CAD build for the part. Positions are in the model's coordinates, mm. A direction names the side the tool comes from. Coordinates: 2 decimals unless noted, no trailing zeros. Order: outer loops, then holes, each group sorted by start corner. A loop starts at its lowest first (then second) coordinate and runs counter-clockwise, first axis right, second up. Notation, with made-up numbers: M 33.25,-30.75 L 79.25,-30.75 A20 ccw 79.25,0.25 Z; hole C 48.5,26.5 d4. An arc over 180 degrees is marked long. One line per item, written item: value.
from build123d import *

# Parameters (mm, degrees)
BOSS_EXTRUDE1_DEPTH     = 100
BOSS_EXTRUDE2_DEPTH     = 100
CUT_EXTRUDE1_DEPTH      = 10
CHAMFER1_SIZE           = 5.5
CHAMFER2_SIZE           = 4
SKETCH8_R               = 2
BOSS_EXTRUDE3_DEPTH     = 9.3
CUT_EXTRUDE3_DEPTH      = 125.214315536
CUT_EXTRUDE3_DEPTH_BACK = 10
SKETCH9_W               = 11
SKETCH9_H               = 9.3
CHAMFER3_SIZE           = 4
CHAMFER4_SIZE           = 3
CHAMFER5_SIZE           = 3
SKETCH10_W              = 5
SKETCH10_H              = 10
CUT_EXTRUDE4_DEPTH      = 94
CHAMFER7_SIZE           = 1
CHAMFER8_SIZE           = 1
SKETCH11_R              = 2.05
CUT_EXTRUDE5_DEPTH      = 10
CHAMFER9_SIZE           = 0.5
SKETCH12_R              = 2
CUT_EXTRUDE6_DEPTH      = 15
SKETCH20_W              = 62.3
SKETCH20_H              = 63.674798271
CUT_EXTRUDE14_DEPTH     = 15
BOSS_EXTRUDE4_DEPTH     = 6
SKETCH22_R              = 2
CUT_EXTRUDE15_DEPTH     = 10
CHAMFER10_SIZE          = 1
CHAMFER10_SIZE2         = 0.414213562
CHAMFER11_SIZE          = 1
CHAMFER11_SIZE2         = 0.414213562


with BuildPart() as part:
    # Sketch4 → Boss-Extrude1 (new body)
    with BuildSketch(Plane.XY):
        Polygon((-18.358738987, 4.974798271), (-27, 4.974798271), (-27, -6.2), (27, -6.2), (27, 4.974798271), (18.358738987, 4.974798271), (21.346410162, -0.2), (-21.346410162, -0.2), align=None)
    extrude(amount=BOSS_EXTRUDE1_DEPTH)

    # Sketch6 → Boss-Extrude2 (add)
    with BuildSketch(Plane.XY.offset(100)):
        Polygon((-24.15, 4.974798271), (-24.15, 52.474798271), (-5.5, 52.474798271), (-5.5, 57.474798271), (-31.15, 57.474798271), (-31.15, -6.2), (-24.15, -6.2), align=None)
        Polygon((24.15, -6.2), (24.15, 52.474798271), (5.5, 52.474798271), (5.5, 57.474798271), (31.15, 57.474798271), (31.15, -6.2), align=None)
    extrude(amount=-BOSS_EXTRUDE2_DEPTH)

    # Sketch7 → Cut-Extrude1 (cut)
    with BuildSketch(Plane(origin=(31.15, 0, 0), x_dir=(0, 0, -1), z_dir=(1, 0, 0))):
        Polygon((-85, 28.724798271), (-81.5, 25.224798271), (-13.5, 25.224798271), (-10, 28.724798271), (-13.5, 32.224798271), (-81.5, 32.224798271), align=None)
    extrude(amount=-CUT_EXTRUDE1_DEPTH, mode=Mode.SUBTRACT)

    # Chamfer1
    chamfer1_edges = [part.edges().sort_by_distance(p)[0] for p in [
        (-24.15, 52.474798271, 50),
        (-24.15, 4.974798271, 50),
        (24.15, 4.974798271, 50),
        (24.15, 52.474798271, 50),
    ]]
    chamfer(chamfer1_edges, length=CHAMFER1_SIZE)

    # Chamfer2
    chamfer2_edges = [part.edges().sort_by_distance(p)[0] for p in [
        (-5.5, 52.474798271, 50),
        (5.5, 52.474798271, 50),
    ]]
    chamfer(chamfer2_edges, length=CHAMFER2_SIZE)

    # Sketch8 → Boss-Extrude3 (add)
    with BuildSketch(Plane(origin=(0, 57.474798271, 0), x_dir=(1, 0, 0), z_dir=(0, 1, 0))):
        Polygon((-21.8, -70), (13.8, -70), (21.8, -62), (21.8, -14), (13.8, -6), (-21.8, -6), align=None)
        with Locations(Location((9.8, -62, 0), (0, 0, 270))):
            Circle(SKETCH8_R, mode=Mode.SUBTRACT)
        with Locations(Location((11.8, -14, 0), (0, 0, 270))):
            Circle(SKETCH8_R, mode=Mode.SUBTRACT)
        with Locations(Location((-11.8, -14, 0), (0, 0, 270))):
            Circle(SKETCH8_R, mode=Mode.SUBTRACT)
        with Locations(Location((-9.8, -62, 0), (0, 0, 270))):
            Circle(SKETCH8_R, mode=Mode.SUBTRACT)
    extrude(amount=BOSS_EXTRUDE3_DEPTH)

    # Sketch9 → Cut-Extrude3 (cut, two sides: drawn at the far end of the back side and taken through both)
    with BuildSketch(Plane.XY.offset(-CUT_EXTRUDE3_DEPTH_BACK)):
        with Locations((0, 62.124798271)):
            Rectangle(SKETCH9_W, SKETCH9_H)
    extrude(amount=CUT_EXTRUDE3_DEPTH + CUT_EXTRUDE3_DEPTH_BACK, mode=Mode.SUBTRACT)

    # Chamfer3
    chamfer3_edges = [part.edges().sort_by_distance(p)[0] for p in [
        (-31.15, -6.2, 50),
        (-31.15, 57.474798271, 50),
        (31.15, -6.2, 50),
        (31.15, 57.474798271, 50),
    ]]
    chamfer(chamfer3_edges, length=CHAMFER3_SIZE)

    # Chamfer4
    chamfer4_edges = [part.edges().sort_by_distance(p)[0] for p in [
        (9.65, 57.474798271, 70),
        (-21.8, 57.474798271, 38),
        (-13.65, 57.474798271, 70),
        (17.8, 57.474798271, 66),
        (21.8, 57.474798271, 38),
        (17.8, 57.474798271, 10),
        (9.65, 57.474798271, 6),
        (-13.65, 57.474798271, 6),
    ]]
    chamfer(chamfer4_edges, length=CHAMFER4_SIZE)

    # Chamfer5
    # the kernel refuses this chamfer: 3 mm, written as the material it adds along each edge
    with BuildSketch(Plane(origin=(31.15, 25.224798271, 81.5), x_dir=(0, -0.014760203742521738, -0.9998910622590239), z_dir=(-1, 0, 0)), Plane(origin=(31.15, 32.224798271, 81.5), x_dir=(0, -0.6965927104131427, 0.7174667907292097), z_dir=(-1, 0, 0))) as chamfer5_piece_1:
        Polygon((CHAMFER5_SIZE * 0.999891062259, -CHAMFER5_SIZE * 0.0147602037425), (-CHAMFER5_SIZE * 0.717466790729, -CHAMFER5_SIZE * 0.696592710413), (0, 0), align=None)
    extrude(amount=7)
    with BuildSketch(Plane(origin=(31.15, 28.724798271, 85), x_dir=(0, 0.7262819568766863, -0.687396915264661), z_dir=(-1, 0, 0))) as chamfer5_piece_2:
        Polygon((CHAMFER5_SIZE * 0.999621916911, CHAMFER5_SIZE * 0.0274958766106), (-CHAMFER5_SIZE * 0.0274958766106, CHAMFER5_SIZE * 0.999621916911), (0, 0), align=None)
    extrude(amount=7)

    # Sketch10 → Cut-Extrude4 (cut)
    with BuildSketch(Plane.XY.offset(100)):
        with Locations((-24.15, 28.724798271)):
            Rectangle(SKETCH10_W, SKETCH10_H)
    extrude(amount=-CUT_EXTRUDE4_DEPTH, mode=Mode.SUBTRACT)

    # Chamfer7
    chamfer7_edges = [part.edges().sort_by_distance(p)[0] for p in [
        (-24.15, 28.724798271, 6),
    ]]
    chamfer(chamfer7_edges, length=CHAMFER7_SIZE)

    # Chamfer8
    chamfer8_edges = [part.edges().sort_by_distance(p)[0] for p in [
        (-24.15, 23.724798271, 52.5),
        (-24.15, 33.724798271, 52.5),
    ]]
    chamfer(chamfer8_edges, length=CHAMFER8_SIZE)

    # Sketch11 → Cut-Extrude5 (cut)
    with BuildSketch(Plane(origin=(0, 66.774798271, 0), x_dir=(1, 0, 0), z_dir=(0, 1, 0))):
        with Locations(Location((-11.8, -14, 0), (0, 0, 270))):
            Circle(SKETCH11_R)
        with Locations(Location((11.8, -14, 0), (0, 0, 270))):
            Circle(SKETCH11_R)
        with Locations(Location((-9.8, -62, 0), (0, 0, 270))):
            Circle(SKETCH11_R)
        with Locations(Location((9.8, -62, 0), (0, 0, 270))):
            Circle(SKETCH11_R)
    extrude(amount=-CUT_EXTRUDE5_DEPTH, mode=Mode.SUBTRACT)

    # Chamfer9
    chamfer9_edges = [part.edges().sort_by_distance(p)[0] for p in [
        (11.8, 66.774798271, 11.95),
        (-9.8, 66.774798271, 59.95),
        (9.8, 66.774798271, 59.95),
        (-11.8, 66.774798271, 11.95),
    ]]
    chamfer(chamfer9_edges, length=CHAMFER9_SIZE)

    # Sketch12 → Cut-Extrude6 (cut)
    with BuildSketch(Plane.XY):
        with Locations((-25, 52.724798271)):
            Circle(SKETCH12_R)
        with Locations((25, 52.724798271)):
            Circle(SKETCH12_R)
        with Locations((-25, 2.724798271)):
            Circle(SKETCH12_R)
        with Locations((25, 2.724798271)):
            Circle(SKETCH12_R)
    extrude(amount=CUT_EXTRUDE6_DEPTH, mode=Mode.SUBTRACT)

    # Sketch20 → Cut-Extrude14 (cut)
    with BuildSketch(Plane.XY.offset(100)):
        with Locations((0, 25.637399136)):
            Rectangle(SKETCH20_W, SKETCH20_H)
    extrude(amount=-CUT_EXTRUDE14_DEPTH, mode=Mode.SUBTRACT)

    # Sketch21 → Boss-Extrude4 (add)
    with BuildSketch(Plane.XY.offset(85)):
        Polygon((-31.15, 11.971631471), (-41.05, 17.687399136), (-41.05, 33.587399136), (-31.15, 39.303166801), align=None)
        Polygon((-13.665767665, -6.2), (-7.95, -16.1), (7.95, -16.1), (13.665767665, -6.2), align=None)
    extrude(amount=-BOSS_EXTRUDE4_DEPTH)

    # Sketch22 → Cut-Extrude15 (cut)
    with BuildSketch(Plane.XY.offset(85)):
        with Locations((-36.15, 25.637399136)):
            Circle(SKETCH22_R)
        with Locations((0, -11.2)):
            Circle(SKETCH22_R)
    extrude(amount=-CUT_EXTRUDE15_DEPTH, mode=Mode.SUBTRACT)

    # Chamfer10
    chamfer10_edges = [part.edges().sort_by_distance(p)[0] for p in [
        (0, -6.2, 79),
    ]]
    chamfer10_side = [part.faces().sort_by_distance(p)[0] for p in [
        (-10.556136515, -11.004653619, 79),
    ]]
    chamfer(chamfer10_edges, length=CHAMFER10_SIZE, length2=CHAMFER10_SIZE2, reference=chamfer10_side[0])

    # Chamfer11
    chamfer11_edges = [part.edges().sort_by_distance(p)[0] for p in [
        (-31.15, 25.637399136, 79),
    ]]
    chamfer11_side = [part.faces().sort_by_distance(p)[0] for p in [
        (-35.954653619, 15.08126262, 79),
    ]]
    chamfer(chamfer11_edges, length=CHAMFER11_SIZE, length2=CHAMFER11_SIZE2, reference=chamfer11_side[0])


solid = part.part
Q1. Which spindle directions (+Z, -Z, +X, -X, +Y, -Y) get a long thin tool onto all of the face, cutting with end or side? Do faces 4 (the face through (7.528, 54.447, 43.095)), 5 (the face through (-26.59, 51.51, 7.4)), 6 (the face through (-9.71, 61.59, 59.95)). Say none if no direction does.
Recorded:
face 4: +Z, -Z
face 5: -Z
face 6: +Y
Q2. Drill centre lines: line 1 along Y through (x, z) = (8.5, 51); line 2 along Y through (x, z) = (25, 6.5); line 3 along X through (y, z) = (33, 67.5). Where is each one in solid material? Low to high.
Recorded:
line 1: y = -6.2 to -0.2, 53.47 to 66.77
line 2: y = -6.2 to 0.72, 4.72 to 50.72, 54.72 to 57.47
line 3: x = -31.15 to -26.65, 24.15 to 31.15
Q3. Slice it at B-B (y = 8.5). List the corners of the cut face in (x, z).
Recorded:
outline: M -31.15,0 L -22.18,0 L -22.18,85 L -31.15,85 Z; M 22.18,0 L 31.15,0 L 31.15,85 L 22.18,85 Z
Q4. Slice it at C-C (x = -36.15). List the corners of the cut face in (y, z).
Recorded:
outline: M 14.86,79 L 23.64,79 L 23.64,85 L 14.86,85 Z; M 27.64,79 L 36.42,79 L 36.42,85 L 27.64,85 Z
Q5. Pin check, flat tips, straight feed: pin 1 Ø8 at (x, z) = (3, 33.5) entering from -Y; pin 2 Ø3 at (x, y) = (8.5, 62.5) entering from +Z; pin 3 Ø8 at (y, z) = (26, 53) entering from -X; pin 4 Ø2 at (x, y) = (-21.5, 27) entering from +Z. Stop position of each tip, or through.
Recorded:
pin 1: stops at y = -6.2
pin 2: stops at z = 70
pin 3: stops at x = -31.15
pin 4: passes through
Q6. Slice it at A-A (x = 0). List the corners of the cut face in (y, z).
Recorded:
outline: M -16.1,79 L -13.2,79 L -13.2,85 L -16.1,85 Z; M -9.2,79 L -7.2,79 L -6.2,78.59 L -6.2,0 L -0.2,0 L -0.2,85 L -9.2,85 Z
Q7. Mould opens along Z. For faces 1 (the face through (10, 56.775, 62)), 2 (the face through (-25, 57.475, 55)), 3 (the face through (18.914, 58.996, 9.022)) say: released by +Z, released by -Z, zero draft, split by the parting line, or undercut.
Recorded:
face 1: undercut
face 2: zero draft
face 3: released by -Z
